Input: part model. Units: mm. Frame: model coordinates. Face numbers are marked on the shaded views. A direction names the side the tool comes from. Round coordinates to 2 decimals unless told otherwise and drop trailing zeros. Loops run counter-clockwise (first coordinate to the right, second up) from the corner with the lowest first, then second, coordinate; pieces in that order, holes last.
1) Section B-B, the plane z = 57. Return loops of the section in (x, y), and give its area (3 significant figures).
2) Ray query, line 1 along Z through (x, y) = (9.6, 0); line 2 along Z through (x, y) = (9.75, -1); line 3 along Z through (x, y) = (10, 8). Return the intervals inside material, ascending.
3) Draft query along X for the marked faces 4 and 5. Return one class per face: pulls with the +X half, pulls with the -X half, needs draft (parallel to the pull), parting line crosses it, or undercut.
4) Section A-A, the plane z = 28. Return loops of the section in (x, y).
5) First-contact query: pin 1 (5 mm diameter, centred on x = 0, z = 28.5, fed in from +Y); pin 2 (13 mm diameter, centred on y = 0, z = 0, fed in from -X); pin 3 (1 mm diameter, centred on y = 2.5, z = 60, fed in from +X). Flat tips, straight axial feed; report the tip coordinate or a pass-through.
6) Access query for the marked faces 1, 2 and 3. Directions: +Z, -Z, +X, -X, +Y, -Y. A direction counts if a zero-diameter tool reaches every point of the face in a straight line with its end or side. Return the directions, or none.
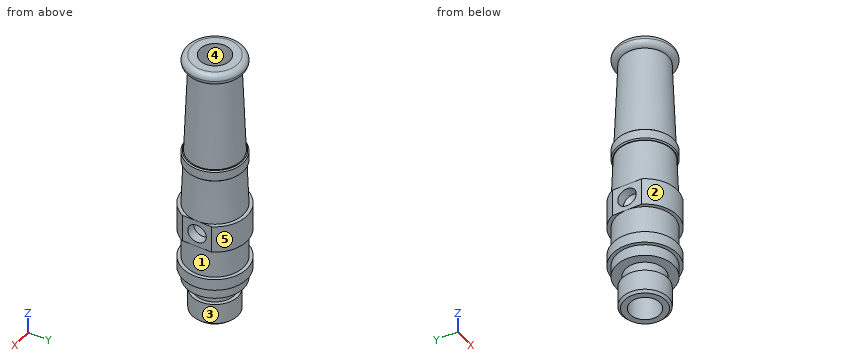
Autodesk Inventor part; units mm, degrees
ref_plane "YZ Plane" through (0, 0, 0) normal (1, 0, 0) x (0, 1, 0)
ref_plane "XZ Plane" through (0, 0, 0) normal (0, 1, 0) x (-1, 0, 0)
ref_plane "XY Plane" through (0, 0, 0) normal (0, 0, 1) x (1, 0, 0)
sketch "草圖1" plane through (0, 0, 0) normal (1, 0, 0) x (0, 1, 0)
  line L0 (0, 0) -> (0, 6)
  line L1 (0, 6) -> (-14, 6)
  line L2 (-14, 6) -> (-14, -6)
  line L3 (-14, -6) -> (0, -6)
  line L4 (0, -6) -> (0, 0)
  line L5 (0, -6) -> (-12.5, -6)
  line L6 (-12.5, -6) -> (-12.5, -19)
  line L7 (-12.5, -19) -> (0, -19)
  line L8 (0, -19) -> (0, -6)
  line L9 (0, -19) -> (-14, -19)
  line L10 (-14, -19) -> (-14, -24)
  line L11 (-14, -24) -> (0, -24)
  line L12 (0, -24) -> (0, -19)
  line L13 (0, -24) -> (-12.5, -24)
  line L14 (-12.5, -24) -> (-12.5, -29)
  line L15 (-12.5, -29) -> (0, -29)
  line L16 (0, -29) -> (0, -24)
  line L17 (0, -29) -> (-8.5, -29)
  line L18 (-8.5, -29) -> (-8.5, -34)
  line L19 (-8.5, -34) -> (0, -34)
  line L20 (0, -34) -> (0, -29)
  line L21 (0, -34) -> (-10, -34)
  line L22 (-10, -34) -> (-10, -44)
  line L23 (-10, -44) -> (0, -44)
  line L24 (0, -44) -> (0, -34)
  line L25 (0, 6) -> (0, 26)
  line L26 (0, 26) -> (-12.5, 26)
  line L27 (-12.5, 26) -> (-12.5, 31)
  line L28 (-12.5, 31) -> (0, 31)
  line L29 (0, 31) -> (0, 26)
  line L30 (0, 31) -> (0, 71)
  line L31 (0, 71) -> (-12.5, 71)
  line L32 (-12.5, 71) -> (-12.5, 76)
  line L33 (-12.5, 76) -> (0, 76)
  line L34 (0, 76) -> (0, 71)
  line L35 (-12.5, 6) -> (-10, 71)
  point P0 (-11.5385, 31)
  point P1 (-11.7308, 26)
  dimension "d0" = 6
  dimension "d1" = 14
  dimension "d3" = 12
  dimension "d5" = 12.5
  dimension "d6" = 13
  dimension "d7" = 14
  dimension "d8" = 5
  dimension "d9" = 12.5
  dimension "d10" = 5
  dimension "d11" = 8.5
  dimension "d12" = 5
  dimension "d13" = 10
  dimension "d14" = 10
  dimension "d15" = 20
  dimension "d16" = 12.5
  dimension "d17" = 5
  dimension "d18" = 40
  dimension "d19" = 12.5
  dimension "d20" = 5
  dimension "d21" = 10
  dimension "d22" = 12.5
revolve "迴轉1" add sketch "草圖1" angle 360 about axis through (0, 0, 31) along (0, 0, 1)
chamfer "倒角1" distance 1 angle 45 1 edges at (0, 10, -44)
chamfer "倒角2" distance 0.5 angle 45 2 edges at (0, 12.5, 26) (0, 12.5, 31)
fillet "圓角1" radius 2.5 2 edges at (0, 12.5, 71) (0, 12.5, 76)
sketch "草圖2" plane through (0, 0, 76) normal (0, 0, 1) x (1, 0, 0)
  circle A0 centre (0, 0) radius 11.5385
  circle A1 centre (0, 0) radius 6.5
  dimension "d31" = 13
extrude "擠出1" cut sketch "草圖2" against normal through all contours A1
thread "螺紋1"
sketch "草圖3" plane through (0, 0, 76) normal (0, 0, 1) x (1, 0, 0)
  line L0 (0, 31.2369) -> (12.5, 31.2369)
  line L1 (12.5, 31.2369) -> (12.5, -26.971)
  line L2 (12.5, -26.971) -> (42.2195, -26.971)
  line L3 (42.2195, -26.971) -> (42.2195, 31.8991)
  line L4 (42.2195, 31.8991) -> (12.5, 31.2369)
  line L5 (0, 31.2369) -> (-12.5, 31.2369)
  line L6 (-12.5, 31.2369) -> (-12.5, -26.3803)
  line L7 (-12.5, -26.3803) -> (-38.1355, -26.3803)
  line L8 (-38.1355, -26.3803) -> (-38.1355, 30.1085)
  line L9 (-38.1355, 30.1085) -> (-12.5, 31.2369)
  point P0 (0, 0)
  dimension "d36" = 12.5
  dimension "d37" = 90
  dimension "d38" = 12.5
extrude "擠出2" cut sketch "草圖3" against normal blind 91.75
sketch "草圖4" plane through (12.5, -6.3048, -6) normal (1, 0, 0) x (0, 0, -1)
  circle A0 centre (-6, 6.3048) radius 4
  dimension "d41" = 8
hole "孔1" at (12.5, 0, 0) direction (-1, 0, 0) diameter 8 depth 4 tip angle 118
mirror "鏡射1" about plane through (0, 0, 0) normal (1, 0, 0) of "孔1"
properties part number "1. 砲管"
Final values:
1. outline: circle Ø21.08 at (0, 0); hole circle Ø13 at (0, 0)
1. area: 216 mm2
2. line 1: z = -43.4 to -34, -29 to -4, 4 to 76
2. line 2: z = -43.2 to -34, -29 to -3.87, 3.87 to 76
2. line 3: z = -24 to -19, -6 to 6
3. face 4: undercut
3. face 5: parting line crosses it
4. outline: circle Ø25 at (0, 0); hole circle Ø13 at (0, 0)
5. pin 1: stops at y = 12.5
5. pin 2: stops at x = -12.5
5. pin 3: stops at x = 10.23
6. face 1: none
6. face 2: +Z, -Z, -Y
6. face 3: -Z
